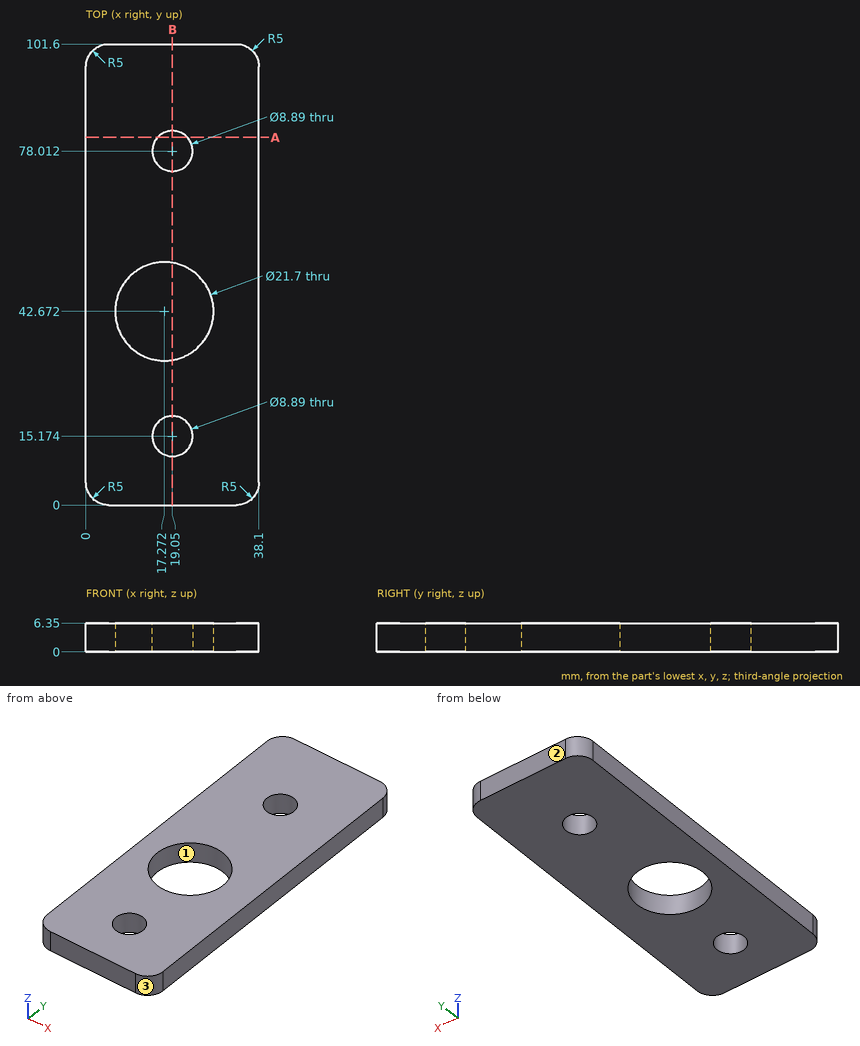
Verification items for this drawing (mm, ordinates from the low corner). Coordinates: 2 decimals unless noted, no trailing zeros. Order: outer loops, then holes, each group sorted by start corner. A loop starts at its lowest first (then second) coordinate and runs counter-clockwise, first axis right, second up.
Q1. Thickness scan on probe 1 along Y at (x, z) = (19.5, 3.5) (1 decimal); probe 2 along Y at (x, z) = (20.5, 4.5) (1 decimal); probe 3 along X at (y, z) = (16, 4). Record the ranges inside material, lowest first.
Reply:
probe 1: y = 0 to 10.8, 19.6 to 32.1, 53.3 to 73.6, 82.4 to 101.6
probe 2: y = 0 to 11, 19.4 to 32.3, 53 to 73.8, 82.2 to 101.6
probe 3: x = 0 to 14.68, 23.42 to 38.1
Q2. Sectioned sample at B-B on x = 19.05. Give the number of separate pieces and of enclosed holes in the cut face, and give its area (3 significant figures).
Reply:
separate pieces: 4
enclosed holes: 0
area: 396 mm2
Q3. Depth check by flat-ended pin: pin 1 Ø8 at (x, y) = (19.05, 78.01) entering from +Z; pin 2 Ø1.5 at (x, y) = (25, 14) entering from -Z. Enter the tip coordinate at first touch or a pass-through.
Reply:
pin 1: passes through
pin 2: stops at z = 0
Q4. Draft check along Y on the marked faces 1, 2 and 3. Enter one of: released by +Y, released by -Y, zero draft, split by the parting line, or undercut.
Reply:
face 1: undercut
face 2: released by +Y
face 3: released by -Y
Q5. Sectioned sample at A-A on y = 81. Record the cut outline in (x, z), and give its area (3 significant figures).
Reply:
outline: (0, 0) - (15.76, 0) - (15.76, 6.35) - (0, 6.35) - close; (22.34, 0) - (38.1, 0) - (38.1, 6.35) - (22.34, 6.35) - close
area: 200 mm2
